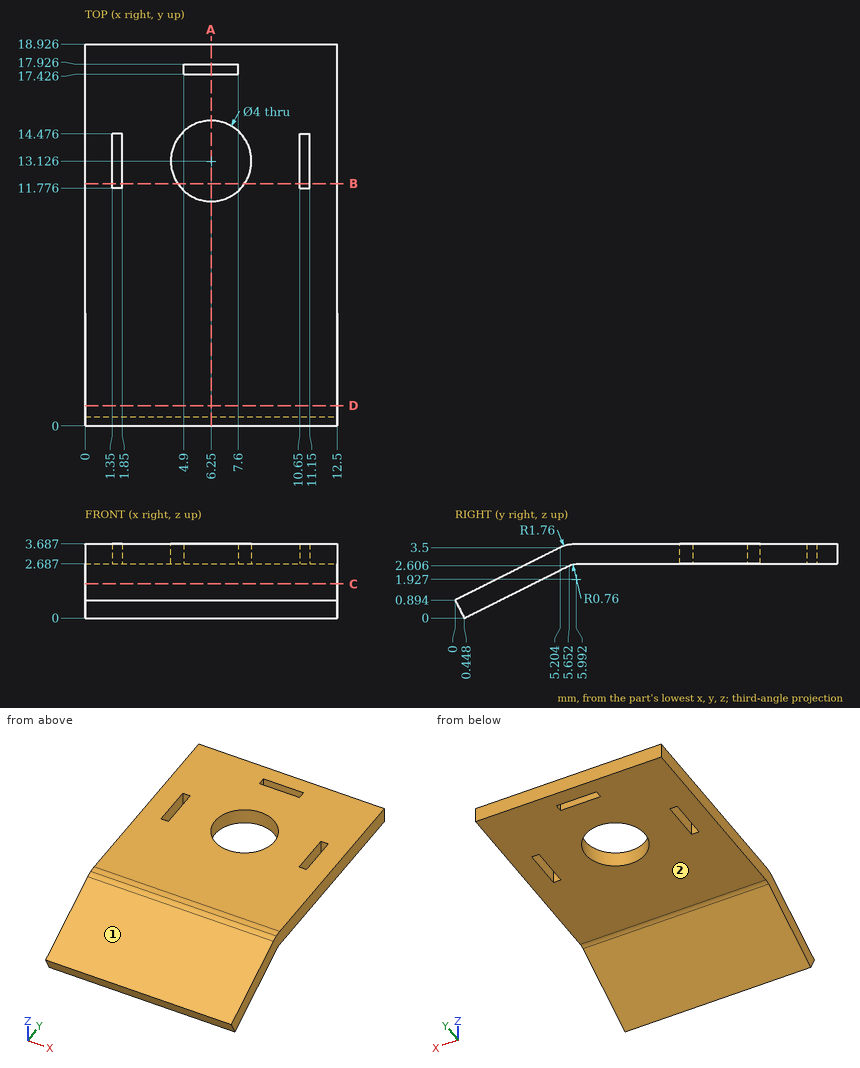
Design review of the part shown in the three views and the two pictorial views. Dimensions are in mm from the part's minimum x, y and z. A direction names the side the tool comes from. Round coordinates to 2 decimals unless told otherwise and drop trailing zeros. Write each loop counter-clockwise with the first axis right and the second up, starting at its lowest first coordinate (ties: lowest second). Pieces come first, ordered by that corner, then holes.
Item 1: We need section C-C on z = 1.7. Write out the cut boundary in (x, y), and give its area (3 significant figures).
Item 2: Clearance check with flat-ended pins moving along their axes: pin 1 Ø0.5 at (x, z) = (6, 3.5) entering from -Y (1 decimal); pin 2 Ø1.5 at (x, z) = (11, 2.5) entering from -Y; pin 3 Ø6 at (x, y) = (7, 10.5) entering from -Z. State where each tip first meets the part, or that it passes through.
Item 3: For probe 1 along Y at (x, z) = (6.25, 3.45) (1 decimal); probe 2 along Y at (x, z) = (6.25, 3.3) (1 decimal); probe 3 along X at (y, z) = (17.5, 2.85), list the stretches that pass through material, from the lowest coordinate up.
Item 4: For the marked faces 1 and 2, list the 3-axis set-ups (+Z, -Z, +X, -X, +Y, -Y) from which the entire face can be reached by the end or side of a thin tool; tool diameter is ignored.
Item 5: We need section A-A on x = 6.25. State how many separate pieces and enclosed holes the cut face has.
Item 6: We need section B-B on y = 12. Write out the cut boundary in (x, z).
Item 7: We need section D-D on y = 1. Write out the cut boundary in (x, z) (1 decimal), and give its area (3 significant figures).
Returned:
1. outline: (0, 1.61) - (12.5, 1.61) - (12.5, 3.84) - (0, 3.84) - close
1. area: 27.9 mm2
2. pin 1: stops at y = 4.7
2. pin 2: stops at y = 1.71
2. pin 3: stops at z = 2.69
3. probe 1: y = 5.1 to 11.1, 15.1 to 17.4, 17.9 to 18.9
3. probe 2: y = 4.8 to 11.1, 15.1 to 17.4, 17.9 to 18.9
3. probe 3: x = 0 to 4.9, 7.6 to 12.5
4. face 1: +Z, +X, -X, -Y
4. face 2: -Z, +X, -X, +Y
5. separate pieces: 3
5. enclosed holes: 0
6. outline: (0, 2.69) - (1.35, 2.69) - (1.35, 3.69) - (0, 3.69) - close; (1.85, 2.69) - (4.6, 2.69) - (4.6, 3.69) - (1.85, 3.69) - close; (7.9, 2.69) - (10.65, 2.69) - (10.65, 3.69) - (7.9, 3.69) - close; (11.15, 2.69) - (12.5, 2.69) - (12.5, 3.69) - (11.15, 3.69) - close
7. outline: (0, 0.3) - (12.5, 0.3) - (12.5, 1.4) - (0, 1.4) - close
7. area: 14.0 mm2
